Verification items for the finished model (mm, model axes). A direction names the side the tool comes from. Coordinates: 2 decimals unless noted, no trailing zeros. Loops run counter-clockwise (first coordinate to the right, second up) from the corner with the lowest first, then second, coordinate; pieces in that order, holes last.
Q1. Sectioned sample at D-D (x = 14.75). Enter the section's corners in (y, z), then the cut area to 3 significant figures.
Q2. Mould release check, pull along X, two halves, no side actions. Record for faces 1 (the face through (3, 1, 11)), 2 (the face through (13.866, 1.014, 0.244)), 3 (the face through (18.631, 9.021, -19.542)), 4 (the face through (9, 0, 0)): +X half, -X half, draft (parallel to the pull), parting line (faces both ways), or undercut.
Q3. Sectioned sample at C-C (y = 7.5). Enter the section's corners in (x, z), then the cut area to 3 significant figures.
Q4. Material ranges on probe 1 along Z at (x, y) = (8.5, 5); probe 2 along Y at (x, z) = (4, -1); probe 3 along Z at (x, y) = (11, 4.25), recorded low to high.
Q5. Sectioned sample at A-A (y = 4). Enter the section's corners in (x, z), then the cut area to 3 significant figures.
Q6. Go/stop test with flat-tipped pins: P1, Ø1.6, axis at y = 5, z = -17, coming from the +X side; P2, Ø1, axis at x = 17, z = -2.5, coming from the +Y side; P3, Ø6, axis at x = 5.5, z = 0.5, coming from the +Y side. Record where each tip stops, or that it passes through.
Q7. Sectioned sample at B-B (z = 0). Enter the section's corners in (x, y), then the cut area to 3 significant figures.
Q8. Access from +Z, -Z, +X, -X, +Y, -Y to the whole of each face (thin tool, end or side, straight path). Record for faces 5 (the face through (20.849, 1.159, 17.156)), 6 (the face through (3.4, 0.99, 13.03)), 7 (the face through (16, 4, 0)).
```python
from build123d import *

# Parameters (mm, degrees)
SKETCH2_W                = 42.3
SKETCH2_H                = 42.3
BOSS_EXTRUDE1_DEPTH      = 12
SKETCH5_R                = 29.910616844
SKETCH5_R_2              = 27
CUT_EXTRUDE4_DEPTH       = 13
CUT_EXTRUDE5_DEPTH       = 10
CUT_EXTRUDE6_DEPTH       = 1.5
BOSS_EXTRUDE2_DEPTH      = 4.5
SKETCH13_W               = 22.65
SKETCH13_H               = 42.3
CUT_EXTRUDE9_DEPTH       = 13
CHAMFER4_SIZE            = 1
CUT_EXTRUDE8_DEPTH       = 3
FILLET12_R               = 1
SKETCH14_R               = 1.75
CUT_EXTRUDE10_DEPTH      = 1
CUT_EXTRUDE10_DEPTH_BACK = 20.65
SKETCH15_R               = 3
CUT_EXTRUDE11_DEPTH      = 4


with BuildPart() as part:
    # Sketch2 → Boss-Extrude1 (new body)
    with BuildSketch(Plane(origin=(0, 0, 0), x_dir=(1, 0, 0), z_dir=(0, 1, 0))):
        Rectangle(SKETCH2_W, SKETCH2_H)
    extrude(amount=BOSS_EXTRUDE1_DEPTH)

    # Sketch5 → Cut-Extrude4 (cut, through all)
    with BuildSketch(Plane(origin=(0, 12, 0), x_dir=(1, 0, 0), z_dir=(0, 1, 0))):
        Circle(SKETCH5_R)
        Circle(SKETCH5_R_2, mode=Mode.SUBTRACT)
    extrude(amount=-CUT_EXTRUDE4_DEPTH, mode=Mode.SUBTRACT)

    # Sketch6 → Cut-Extrude5 (cut)
    with BuildSketch(Plane(origin=(0, 12, 0), x_dir=(1, 0, 0), z_dir=(0, 1, 0))):
        with BuildLine():
            Line((0, 18), (-21.15, 18))
            Line((-21.15, 18), (-21.15, -18))
            Line((-21.15, -18), (0, -18))
            ThreePointArc((0, -18), (18, 0), (0, 18))
        make_face()
    extrude(amount=-CUT_EXTRUDE5_DEPTH, mode=Mode.SUBTRACT)

    # Sketch7 → Cut-Extrude6 (cut)
    with BuildSketch(Plane(origin=(0, 2, 0), x_dir=(1, 0, 0), z_dir=(0, 1, 0))):
        with BuildLine():
            Line((-2, 5.1), (2, 5.1))
            ThreePointArc((2, 5.1), (7.1, 0), (2, -5.1))
            Line((2, -5.1), (-2, -5.1))
            ThreePointArc((-2, -5.1), (-7.1, 0), (-2, 5.1))
        make_face()
    extrude(amount=-CUT_EXTRUDE6_DEPTH, mode=Mode.SUBTRACT)

    # Sketch8 → Boss-Extrude2 (add)
    with BuildSketch(Plane(origin=(0, 2, 0), x_dir=(1, 0, 0), z_dir=(0, 1, 0))):
        with BuildLine():
            Line((0, 16), (-21.15, 16))
            Line((-21.15, 16), (-21.15, 16.783250579))
            ThreePointArc((-21.15, 16.783250579), (-20.646271202, 17.399180597), (-20.124611797, 18))
            Line((-20.124611797, 18), (0, 18))
            ThreePointArc((0, 18), (18, 0), (0, -18))
            Line((0, -18), (-20.124611797, -18))
            ThreePointArc((-20.124611797, -18), (-20.646271202, -17.399180597), (-21.15, -16.783250579))
            Line((-21.15, -16.783250579), (-21.15, -16))
            Line((-21.15, -16), (0, -16))
            ThreePointArc((0, -16), (16, 0), (0, 16))
        make_face()
    extrude(amount=BOSS_EXTRUDE2_DEPTH)

    # Sketch13 → Cut-Extrude9 (cut, through all)
    with BuildSketch(Plane(origin=(0, 12, 0), x_dir=(1, 0, 0), z_dir=(0, 1, 0))):
        with Locations((-9.825, 0)):
            Rectangle(SKETCH13_W, SKETCH13_H)
    extrude(amount=-CUT_EXTRUDE9_DEPTH, mode=Mode.SUBTRACT)

    # Chamfer4
    chamfer4_edges = [part.edges().sort_by_distance(p)[0] for p in [
        (9.14162529, 0, 21.15),
        (21.15, 0, 0),
        (9.14162529, 0, -21.15),
        (19.091883092, 0, -19.091883092),
        (19.091883092, 0, 19.091883092),
    ]]
    chamfer(chamfer4_edges, length=CHAMFER4_SIZE)

    # Sketch11 → Cut-Extrude8 (cut, through all)
    with BuildSketch(Plane(origin=(0, 2, 0), x_dir=(1, 0, 0), z_dir=(0, 1, 0))):
        with BuildLine():
            Line((3, 13.539392014), (3, 9.539392014))
            ThreePointArc((3, 9.539392014), (10, 0), (3, -9.539392014))
            Line((3, -9.539392014), (3, -13.539392014))
            ThreePointArc((3, -13.539392014), (13.867773293, 0), (3, 13.539392014))
        make_face()
    extrude(amount=-CUT_EXTRUDE8_DEPTH, mode=Mode.SUBTRACT)

    # Fillet12
    fillet12_edges = [part.edges().sort_by_distance(p)[0] for p in [
        (3, 1, -13.539392014),
        (3, 1, 13.539392014),
        (3, 1, 9.539392014),
        (3, 1, -9.539392014),
    ]]
    fillet(fillet12_edges, radius=FILLET12_R)

    # Sketch14 → Cut-Extrude10 (cut, two sides)
    with BuildSketch(Plane.ZY.offset(-1.5)) as cut_extrude10_sk:
        with Locations((-18.539766161, 4)):
            Circle(SKETCH14_R)
        with Locations((18.539766161, 4)):
            Circle(SKETCH14_R)
    extrude(amount=CUT_EXTRUDE10_DEPTH, mode=Mode.SUBTRACT)
    extrude(cut_extrude10_sk.sketch, amount=-CUT_EXTRUDE10_DEPTH_BACK, mode=Mode.SUBTRACT)

    # Sketch15 → Cut-Extrude11 (cut)
    with BuildSketch(Plane(origin=(21.15, 0, 0), x_dir=(0, 0, -1), z_dir=(1, 0, 0))):
        with Locations((-18.539766161, 4)):
            Circle(SKETCH15_R)
        with Locations((18.539766161, 4)):
            Circle(SKETCH15_R)
    extrude(amount=-CUT_EXTRUDE11_DEPTH, mode=Mode.SUBTRACT)


solid = part.part
```
Geometry check:
1. outline: (0, -20.15) - (1, -21.15) - (12, -21.15) - (12, -10.32) - (6.5, -10.32) - (6.5, -6.2) - (2, -6.2) - (2, 6.2) - (6.5, 6.2) - (6.5, 10.32) - (12, 10.32) - (12, 21.15) - (1, 21.15) - (0, 20.15) - close; hole circle Ø3.5 at (4, -18.54); hole circle Ø3.5 at (4, 18.54)
1. area: 318 mm2
2. face 1: undercut
2. face 2: undercut
2. face 3: +X half
2. face 4: draft
3. outline: (1.5, -21.15) - (16.78, -21.15) arc R27 ccw to (21.15, -16.78) - (21.15, 16.78) arc R27 ccw to (16.78, 21.15) - (1.5, 21.15) - (1.5, 17.94) arc R18 cw to (1.5, -17.94) - close
3. area: 359 mm2
4. probe 1: z = -21.15 to -19.98, -17.1 to -13.56, 13.56 to 17.1, 19.98 to 21.15
4. probe 2: y = 0 to 0.5
4. probe 3: z = -21.15 to -20.27, -16.81 to -11.62, 11.62 to 16.81, 20.27 to 21.15
5. outline: (1.5, -21.15) - (16.78, -21.15) arc R27 ccw to (17.15, -20.85) - (17.15, -20.29) - (1.5, -20.29) - close; (1.5, -16.79) - (17.15, -16.79) - (17.15, -15.54) - (21.15, -15.54) - (21.15, 15.54) - (17.15, 15.54) - (17.15, 16.79) - (1.5, 16.79) - (1.5, 15.93) arc R16 cw to (1.5, -15.93) - close; (1.5, 20.29) - (17.15, 20.29) - (17.15, 20.85) arc R27 ccw to (16.78, 21.15) - (1.5, 21.15) - close
5. area: 322 mm2
6. P1: stops at x = 17.15
6. P2: stops at y = 6.5
6. P3: stops at y = 2
7. outline: (1.5, 0) - (10, 0) - (10, 2) - (7.1, 2) - (7.1, 0.5) - (1.5, 0.5) - close; (13.87, 0) - (20.15, 0) - (21.15, 1) - (21.15, 12) - (18, 12) - (18, 6.5) - (16, 6.5) - (16, 2) - (13.87, 2) - close
7. area: 63.2 mm2
8. face 5: +Z, +X, +Y, -Y
8. face 6: +Y, -Y
8. face 7: -X, +Y
